Here's how the part is built. I have some questions about the finished solid (model axes, mm). Face numbers are marked on the shaded views. A direction names the side the tool comes from. Round coordinates to 2 decimals unless told otherwise and drop trailing zeros. Order: outer loops, then holes, each group sorted by start corner. A loop starts at its lowest first (then second) coordinate and runs counter-clockwise, first axis right, second up. Notation, with made-up numbers: (76.25, -22.5) -> (97.25, -22.5) arc R12 cw to (97.25, -6.5) -> close; hole circle Ø1 at (-4.75, 27.25). An arc over 180 degrees is marked (long way). Use a Markdown table: item, result. Add a question column.
(1) I want a section at D-D, the plane x = -13.5. Please give me the cut outline in (y, z), then the cut area to 3 significant figures.
(2) I want a section at C-C, the plane z = 25.75. Please give me the cut outline in (x, y), then the cut area to 3 significant figures.
(3) If I drill on probe 1 along X at (y, z) = (-7.5, 16); probe 2 along X at (y, z) = (-9.25, 14.75); probe 3 along Z at (x, y) = (-22, -23.5), over which ranges is the centre line in solid material (lowest first)?
(4) I want a section at B-B, the plane y = -16.25. Please give me the cut outline in (x, z), then the cut area to 3 significant figures.
(5) I want a section at A-A, the plane z = 14.25. Please give me the cut outline in (x, y), then the cut area to 3 significant figures.
(6) Thinking about a two-plate mould opening in X: for the marked faces 4, 5 and 6, which applies, pulls with the +X half, pulls with the -X half, needs draft (parallel to the pull), parting line crosses it, or undercut?
(7) I'm going to push flat-ended pins straight in: P1, Ø7.5, axis at x = 42.5, y = -18, coming from the +Z side; P2, Ø2, axis at y = -20, z = 11, coming from the -X side; P3, Ø2, axis at y = -8, z = 8.5, coming from the -X side; P4, Ø3, axis at x = 56.5, y = -16, coming from the +Z side. Where does each tip first touch, or does it pass through?
(8) On a 3-axis mill with a long thin cutter (end or side, diameter ignored), from which of +Z, -Z, +X, -X, +Y, -Y can I reach the whole of each face in a straight line? I mean the marked faces 1, 2 and 3. Say none if no direction works.
from build123d import *

# Parameters (mm, degrees)
F1_DEPTH = 25
F2_R     = 7.5
F3_DEPTH = 25
F4_R     = 5


with BuildPart() as f1:
    # F0 (on Front) → F1 (new body)
    with BuildSketch(Plane.XZ):
        with BuildLine():
            Line((-36.079331, 26.828598), (-42.079331, 26.828598))
            Line((-42.079331, 26.828598), (-42.079331, 11.400025))
            Line((-42.079331, 11.400025), (-36.079331, 11.400025))
            Line((-36.079331, 11.400025), (-1.079331, 11.400025))
            ThreePointArc((-1.079331, 11.400025), (13.879066, 3.078612), (28.837463, 11.400025))
            Line((28.837463, 11.400025), (69.837463, 11.400025))
            Line((69.837463, 11.400025), (69.837463, 26.828598))
            Line((69.837463, 26.828598), (63.837463, 26.828598))
            Line((63.837463, 26.828598), (63.837463, 19.400025))
            Line((63.837463, 19.400025), (28.837463, 19.400025))
            ThreePointArc((28.837463, 19.400025), (13.879066, 9.078612), (-1.079331, 19.400025))
            Line((-1.079331, 19.400025), (-36.079331, 19.400025))
            Line((-36.079331, 19.400025), (-36.079331, 26.828598))
        make_face()
    extrude(amount=F1_DEPTH)

    # F2 (on face) → F3 (cut)
    with BuildSketch(Plane(origin=(0, 0, 11.400025), x_dir=(1, 0, 0), z_dir=(0, 0, -1))):
        with Locations((-23.09421, 11.928692)):
            Circle(F2_R)
        with Locations((52.305905, 11.928692)):
            Circle(F2_R)
    extrude(amount=-F3_DEPTH, mode=Mode.SUBTRACT)

    # F4
    f4_edges = [f1.edges().sort_by_distance(p)[0] for p in [
        (-39.079331, -25, 26.828598),
        (-39.079331, 0, 26.828598),
        (-42.079331, -12.5, 11.400025),
        (69.837463, -12.5, 11.400025),
        (66.837463, -25, 26.828598),
        (66.837463, 0, 26.828598),
        (-1.079331, -12.5, 11.400025),
        (28.837463, -12.5, 11.400025),
        (-42.079331, -12.5, 26.828598),
        (-42.079331, 0, 19.114311),
        (-42.079331, -25, 19.114311),
    ]]
    fillet(f4_edges, radius=F4_R)


solid = f1.part
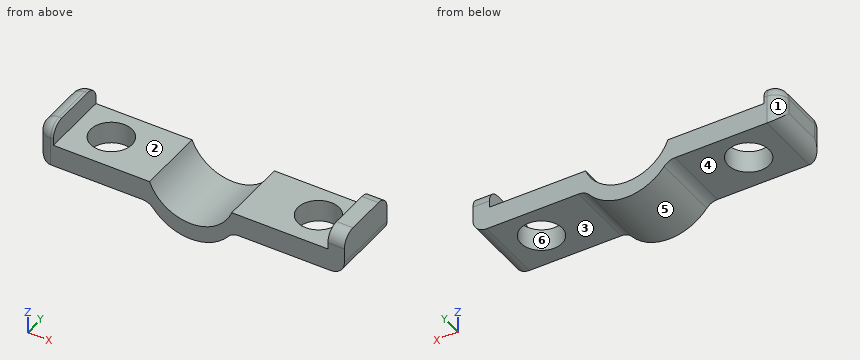
Taken from the geometry:
| question | item | result |
|---|---|---|
| 1 | outline | (-25, 11.4) -> (0, 11.4) -> (0, 19.4) -> (-25, 19.4) -> close |
| 1 | area | 200 mm2 |
| 2 | outline | (-40.18, -20) arc R3.1 ccw to (-37.08, -23.1) -> (-36.08, -23.1) -> (-36.08, -1.9) -> (-37.08, -1.9) arc R3.1 ccw to (-40.18, -5) -> close; (63.84, -23.1) -> (69.84, -23.1) -> (69.84, -1.9) -> (63.84, -1.9) -> close |
| 2 | area | 210 mm2 |
| 3 | probe 1 | x = -42.06 to -29.15, -17.04 to 0.7, 27.05 to 46.25, 58.36 to 69.82 |
| 3 | probe 2 | x = -41.8 to -30.1, -16.09 to 1.66, 26.1 to 45.3, 59.31 to 69.56 |
| 3 | probe 3 | z = 11.4 to 19.4 |
| 4 | outline | (-42.08, 16.4) arc R5 ccw to (-37.08, 11.4) -> (-29.22, 11.4) -> (-29.22, 19.4) -> (-36.08, 19.4) -> (-36.08, 26.83) -> (-37.08, 26.83) arc R5 ccw to (-42.08, 21.83) -> close; (-16.96, 11.4) -> (-3.64, 11.4) arc R5 cw to (0.23, 9.56) arc R17.61 ccw to (27.52, 9.56) arc R5 cw to (31.4, 11.4) -> (46.18, 11.4) -> (46.18, 19.4) -> (28.84, 19.4) arc R16 cw to (-1.08, 19.4) -> (-16.96, 19.4) -> close; (58.44, 11.4) -> (64.84, 11.4) arc R5 ccw to (69.84, 16.4) -> (69.84, 26.83) -> (63.84, 26.83) -> (63.84, 19.4) -> (58.44, 19.4) -> close |
| 4 | area | 726 mm2 |
| 5 | outline | (-41.59, -22.15) arc R5 ccw to (-37.08, -25) -> (2.1, -25) -> (2.1, 0) -> (-37.08, 0) arc R5 ccw to (-41.59, -2.85) -> close; (25.66, -25) -> (69.35, -25) -> (69.35, 0) -> (25.66, 0) -> close; hole circle Ø15 at (-23.09, -11.93); hole circle Ø15 at (52.31, -11.93) |
| 5 | area | 1,820 mm2 |
| 6 | face 4 | needs draft |
| 6 | face 5 | parting line crosses it |
| 6 | face 6 | undercut |
| 7 | P1 | stops at z = 19.4 |
| 7 | P2 | stops at x = -39.45 |
| 7 | P3 | stops at x = 0.28 |
| 7 | P4 | passes through |
| 8 | face 1 | +Z, -Z, -X, +Y |
| 8 | face 2 | +Z, +Y, -Y |
| 8 | face 3 | -Z, +X, +Y, -Y |
